Read the model definition and answer for the solid it produces. Units are mm, in the model's axes. Round coordinates to 2 decimals unless told otherwise and drop trailing zeros. Write each loop counter-clockwise with the first axis right and the second up, starting at its lowest first coordinate (ties: lowest second). Pieces come first, ordered by that corner, then holes. Notation, with made-up numbers: (62.5, 0) -> (98.5, 0) arc R20 cw to (98.5, 29) -> close; hole circle Ø7 at (1, 42.5). An arc over 180 degrees is marked (long way). Return JSON: item names as keys, results as strings.
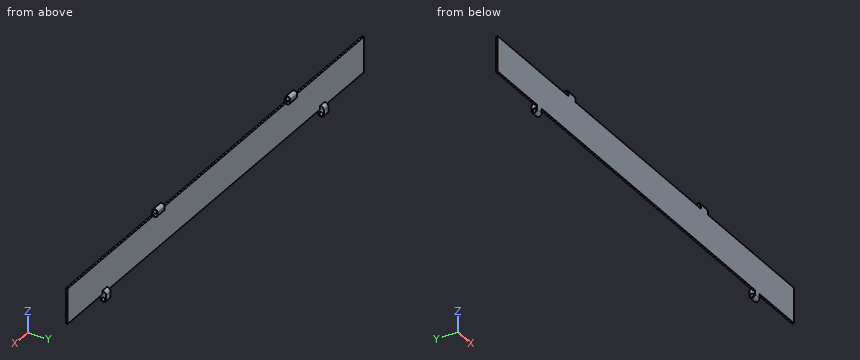
from build123d import *

# Parameters (mm, degrees)
SZKIC1_W                          = 1280
SZKIC1_H                          = 97
DODANIE_WYCI_GNI_CIE1_DEPTH       = 5
DODANIE_WYCI_GNI_CIE2_START       = -5
SZKIC2_W                          = 20
SZKIC2_H                          = 30
DODANIE_WYCI_GNI_CIE2_DEPTH       = 15
ZAOKR_GLENIE2_RADIUS              = 7.5
ZAOKR_GLENIE2_LENGTH              = 20
WYTNIJ_WYCI_GNI_CIE1_REACH        = 1114.213
SZKIC3_R                          = 5
DODANIE_WYCI_GNI_CIE3_START       = -5
SZKIC4_W                          = 30
SZKIC4_H                          = 22.65
DODANIE_WYCI_GNI_CIE3_DEPTH       = 15
ZAOKR_GLENIE3_R                   = 10
ZAOKR_GLENIE4_RADIUS              = 7.5
ZAOKR_GLENIE4_LENGTH              = 30
WYTNIJ_WYCI_GNI_CIE2_REACH        = 979.518
SZKIC5_R                          = 5
SFAZOWANIE1_SIZE                  = 1
ZAOKR_GLENIE5_R                   = 10
ZAOKR_GLENIE4_OF_LUSTRO2_2_RADIUS = 7.5
ZAOKR_GLENIE4_OF_LUSTRO2_2_LENGTH = 30
ZAOKR_GLENIE5_OF_LUSTRO2_R        = 10
ZAOKR_GLENIE2_OF_LUSTRO3_2_RADIUS = 7.5
ZAOKR_GLENIE2_OF_LUSTRO3_2_LENGTH = 20
ZAOKR_GLENIE3_OF_LUSTRO3_R        = 10


with BuildPart() as part:
    # Szkic1 → Dodanie-wyciągnięcie1 (new body)
    with BuildSketch(Plane(origin=(0, 0, 0), x_dir=(1, 0, 0), z_dir=(0, 1, 0))):
        Rectangle(SZKIC1_W, SZKIC1_H)
    extrude(amount=DODANIE_WYCI_GNI_CIE1_DEPTH)

    # Szkic2 → Dodanie-wyciągnięcie2 (add)
    with BuildSketch(Plane(origin=(0, 5, 0), x_dir=(1, 0, 0), z_dir=(0, 1, 0)).offset(DODANIE_WYCI_GNI_CIE2_START)):
        with Locations((-460, 53.5)):
            Rectangle(SZKIC2_W, SZKIC2_H)
    dodanie_wyci_gni_cie2 = extrude(amount=DODANIE_WYCI_GNI_CIE2_DEPTH)

    # Zaokrąglenie2: full round fillet: the end face becomes a half cylinder, R = half its width
    zaokr_glenie2_face = Plane((-460, 7.5, -68.5), x_dir=(-1, 0, 0), z_dir=(0, 0, -1))  # on the end face: x along it, z out of the body
    zaokr_glenie2_slab = zaokr_glenie2_face.offset(-ZAOKR_GLENIE2_RADIUS / 2) * Box(ZAOKR_GLENIE2_LENGTH, 2 * ZAOKR_GLENIE2_RADIUS, ZAOKR_GLENIE2_RADIUS, mode=Mode.PRIVATE)  # the body's end, R deep
    zaokr_glenie2_round = Plane((-460, 7.5, -61), x_dir=(0, 0, -1), z_dir=(-1, 0, 0)) * Cylinder(ZAOKR_GLENIE2_RADIUS, ZAOKR_GLENIE2_LENGTH, mode=Mode.PRIVATE)  # its axis R under the face
    add(zaokr_glenie2_slab - zaokr_glenie2_round, mode=Mode.SUBTRACT)

    # Szkic3 → Wytnij-wyciągnięcie1 (cut, up to next)
    with BuildSketch(Plane.ZY.offset(470), mode=Mode.PRIVATE) as wytnij_wyci_gni_cie1_sk1:
        with Locations((-61, 7.5)):
            Circle(SZKIC3_R)
    wytnij_wyci_gni_cie1_tool1 = extrude(wytnij_wyci_gni_cie1_sk1.sketch, amount=-WYTNIJ_WYCI_GNI_CIE1_REACH, mode=Mode.PRIVATE) & part.part
    wytnij_wyci_gni_cie1 = wytnij_wyci_gni_cie1_tool1.solids().sort_by_distance((-470, 7.5, -61))[0]
    add(wytnij_wyci_gni_cie1, mode=Mode.SUBTRACT)

    # Szkic4 → Dodanie-wyciągnięcie3 (add)
    with BuildSketch(Plane(origin=(0, 5, 0), x_dir=(1, 0, 0), z_dir=(0, 1, 0)).offset(DODANIE_WYCI_GNI_CIE3_START)):
        with Locations((-320, -54.825)):
            Rectangle(SZKIC4_W, SZKIC4_H)
    dodanie_wyci_gni_cie3 = extrude(amount=DODANIE_WYCI_GNI_CIE3_DEPTH)

    # Zaokrąglenie3
    zaokr_glenie3_edges = [part.edges().sort_by_distance(p)[0] for p in [
        (-460, 15, -38.5),
    ]]
    fillet(zaokr_glenie3_edges, radius=ZAOKR_GLENIE3_R - 0.0001)  # a hair under: the kernel refuses the full size

    # Zaokrąglenie4: full round fillet: the end face becomes a half cylinder, R = half its width
    zaokr_glenie4_face = Plane((-320, 7.5, 66.15), x_dir=(1, 0, 0), z_dir=(0, 0, 1))  # on the end face: x along it, z out of the body
    zaokr_glenie4_slab = zaokr_glenie4_face.offset(-ZAOKR_GLENIE4_RADIUS / 2) * Box(ZAOKR_GLENIE4_LENGTH, 2 * ZAOKR_GLENIE4_RADIUS, ZAOKR_GLENIE4_RADIUS, mode=Mode.PRIVATE)  # the body's end, R deep
    zaokr_glenie4_round = Plane((-320, 7.5, 58.65), x_dir=(0, 0, 1), z_dir=(1, 0, 0)) * Cylinder(ZAOKR_GLENIE4_RADIUS, ZAOKR_GLENIE4_LENGTH, mode=Mode.PRIVATE)  # its axis R under the face
    add(zaokr_glenie4_slab - zaokr_glenie4_round, mode=Mode.SUBTRACT)

    # Szkic5 → Wytnij-wyciągnięcie2 (cut, up to next)
    with BuildSketch(Plane.ZY.offset(335), mode=Mode.PRIVATE) as wytnij_wyci_gni_cie2_sk1:
        with Locations((58.65, 7.5)):
            Circle(SZKIC5_R)
    wytnij_wyci_gni_cie2_tool1 = extrude(wytnij_wyci_gni_cie2_sk1.sketch, amount=-WYTNIJ_WYCI_GNI_CIE2_REACH, mode=Mode.PRIVATE) & part.part
    wytnij_wyci_gni_cie2 = wytnij_wyci_gni_cie2_tool1.solids().sort_by_distance((-335, 7.5, 58.65))[0]
    add(wytnij_wyci_gni_cie2, mode=Mode.SUBTRACT)

    # Sfazowanie1
    sfazowanie1_edges = [part.edges().sort_by_distance(p)[0] for p in [
        (-450, 7.5, -66),
        (-470, 7.5, -66),
        (-305, 7.5, 53.65),
        (-335, 7.5, 53.65),
    ]]
    chamfer(sfazowanie1_edges, length=SFAZOWANIE1_SIZE)

    # Zaokrąglenie5
    zaokr_glenie5_edges = [part.edges().sort_by_distance(p)[0] for p in [
        (-320, 15, 43.5),
    ]]
    fillet(zaokr_glenie5_edges, radius=ZAOKR_GLENIE5_R - 0.0001)  # a hair under: the kernel refuses the full size

    # Lustro2: Dodanie-wyciągnięcie3, Wytnij-wyciągnięcie2 across plane
    add(dodanie_wyci_gni_cie3.mirror(Plane(origin=(-34, 0, 0), x_dir=(0, 0, 1), z_dir=(1, 0, 0))))
    add(wytnij_wyci_gni_cie2.mirror(Plane(origin=(-34, 0, 0), x_dir=(0, 0, 1), z_dir=(1, 0, 0))), mode=Mode.SUBTRACT)

    # Zaokrąglenie4 of Lustro2 2: full round fillet: the end face becomes a half cylinder, R = half its width
    zaokr_glenie4_of_lustro2_2_face = Plane((252, 7.5, 66.15), x_dir=(-1, 0, 0), z_dir=(0, 0, 1))  # on the end face: x along it, z out of the body
    zaokr_glenie4_of_lustro2_2_slab = zaokr_glenie4_of_lustro2_2_face.offset(-ZAOKR_GLENIE4_OF_LUSTRO2_2_RADIUS / 2) * Box(ZAOKR_GLENIE4_OF_LUSTRO2_2_LENGTH, 2 * ZAOKR_GLENIE4_OF_LUSTRO2_2_RADIUS, ZAOKR_GLENIE4_OF_LUSTRO2_2_RADIUS, mode=Mode.PRIVATE)  # the body's end, R deep
    zaokr_glenie4_of_lustro2_2_round = Plane((252, 7.5, 58.65), x_dir=(0, 0, 1), z_dir=(-1, 0, 0)) * Cylinder(ZAOKR_GLENIE4_OF_LUSTRO2_2_RADIUS, ZAOKR_GLENIE4_OF_LUSTRO2_2_LENGTH, mode=Mode.PRIVATE)  # its axis R under the face
    add(zaokr_glenie4_of_lustro2_2_slab - zaokr_glenie4_of_lustro2_2_round, mode=Mode.SUBTRACT)

    # Zaokrąglenie5 of Lustro2
    zaokr_glenie5_of_lustro2_edges = [part.edges().sort_by_distance(p)[0] for p in [
        (252, 15, 43.5),
    ]]
    fillet(zaokr_glenie5_of_lustro2_edges, radius=ZAOKR_GLENIE5_OF_LUSTRO2_R - 0.0001)  # a hair under: the kernel refuses the full size

    # Lustro3: Dodanie-wyciągnięcie2, Wytnij-wyciągnięcie1 across plane
    add(dodanie_wyci_gni_cie2.mirror(Plane(origin=(10, 0, 0), x_dir=(0, 0, 1), z_dir=(1, 0, 0))))
    add(wytnij_wyci_gni_cie1.mirror(Plane(origin=(10, 0, 0), x_dir=(0, 0, 1), z_dir=(1, 0, 0))), mode=Mode.SUBTRACT)

    # Zaokrąglenie2 of Lustro3 2: full round fillet: the end face becomes a half cylinder, R = half its width
    zaokr_glenie2_of_lustro3_2_face = Plane((480, 7.5, -68.5), x_dir=(1, 0, 0), z_dir=(0, 0, -1))  # on the end face: x along it, z out of the body
    zaokr_glenie2_of_lustro3_2_slab = zaokr_glenie2_of_lustro3_2_face.offset(-ZAOKR_GLENIE2_OF_LUSTRO3_2_RADIUS / 2) * Box(ZAOKR_GLENIE2_OF_LUSTRO3_2_LENGTH, 2 * ZAOKR_GLENIE2_OF_LUSTRO3_2_RADIUS, ZAOKR_GLENIE2_OF_LUSTRO3_2_RADIUS, mode=Mode.PRIVATE)  # the body's end, R deep
    zaokr_glenie2_of_lustro3_2_round = Plane((480, 7.5, -61), x_dir=(0, 0, -1), z_dir=(1, 0, 0)) * Cylinder(ZAOKR_GLENIE2_OF_LUSTRO3_2_RADIUS, ZAOKR_GLENIE2_OF_LUSTRO3_2_LENGTH, mode=Mode.PRIVATE)  # its axis R under the face
    add(zaokr_glenie2_of_lustro3_2_slab - zaokr_glenie2_of_lustro3_2_round, mode=Mode.SUBTRACT)

    # Zaokrąglenie3 of Lustro3
    zaokr_glenie3_of_lustro3_edges = [part.edges().sort_by_distance(p)[0] for p in [
        (480, 15, -38.5),
    ]]
    fillet(zaokr_glenie3_of_lustro3_edges, radius=ZAOKR_GLENIE3_OF_LUSTRO3_R - 0.0001)  # a hair under: the kernel refuses the full size


solid = part.part
Item 1: Straight lines are drawn through the part: L1, parallel to Y at x = -461, z = -61; L2, parallel to X at y = 14.25, z = -62; L3, parallel to X at y = 6.75, z = 52.5. For each, find the intervals that lie inside material, in ascending order. Write a range as [from, to].
Worked answers:
{"L1": "y = [0, 2.5], [12.5, 15]", "L2": "x = [-470, -450], [470, 490]", "L3": "x = [-335, -305], [237, 267]"}
Item 2: Section A-A (z = -16) is taken. Give the vertices of the cut face in (x, y), then the cut area to 3 significant figures.
Worked answers:
{"outline": "(-640, 0) -> (640, 0) -> (640, 5) -> (-640, 5) -> close", "area": "6,400 mm2"}
Item 3: Section B-B (y = 9.75) is taken. State how many separate pieces and enclosed holes the cut face has, then the cut area to 3 significant figures.
Worked answers:
{"separate pieces": "8", "enclosed holes": "0", "area": "1,510 mm2"}
Item 4: Section C-C (x = -17) is taken. Give the vertices of the cut face in (y, z).
Worked answers:
{"outline": "(0, -48.5) -> (5, -48.5) -> (5, 48.5) -> (0, 48.5) -> close"}
Item 5: Flat-ended cylindrical pins translate along their axes: pin 1 (2.5 mm diameter, centred on x = -588, y = 2.5, fed in from -Z); pin 2 (2.5 mm diameter, centred on x = -411.5, y = 2, fed in from +Z); pin 3 (1.5 mm diameter, centred on x = -382, z = 47.5, fed in from +Y). Find the tip coordinate at first contact, or state that the pin passes through.
Worked answers:
{"pin 1": "stops at z = -48.5", "pin 2": "stops at z = 48.5", "pin 3": "stops at y = 5"}
